Model file for the job. Use its own axes, mm. A direction names the side the tool comes from. Round coordinates to 2 decimals unless told otherwise and drop trailing zeros. Loops run counter-clockwise (first coordinate to the right, second up) from the corner with the lowest first, then second, coordinate; pieces in that order, holes last. Notation, with made-up numbers: (39, 56) -> (44, 56) arc R32 cw to (44, 90) -> close; hole circle Ø11 at (46, 29.5). An arc over 180 degrees is marked (long way). Use a Markdown table: item, result.
Autodesk Fusion 360 part; units mm, degrees
sketch "Sketch1" plane through (0, 0, 0) normal (0, 0, 1) x (1, 0, 0)
  line L0 (33, -21) -> (-33, -21)
  line L1 (-33, -21) -> (-33, 21)
  line L2 (-33, 21) -> (33, 21)
  line L3 (33, 21) -> (33, -21)
  line L4 (33, -21) -> (-33, 21) construction
  line L5 (-33, -21) -> (33, 21) construction
  dimension "d1" = 66
  dimension "d2" = 42
extrude "Extrude1" add sketch "Sketch1" along normal blind 12
chamfer "Chamfer1" distance 12 angle 45 2 edges at (33, -21, 6) (33, 21, 6)
sketch "Sketch2" plane through (0, 0, 12) normal (0, 0, 1) x (-1, 0, 0)
  line L0 (-33, -9) -> (-21, -21)
  line L1 (-21, -21) -> (33, -21)
  line L2 (33, -21) -> (33, 21)
  line L3 (33, 21) -> (-21, 21)
  line L4 (-21, 21) -> (-33, 9)
  line L5 (-33, 9) -> (-33, -9)
  line L6 (33, -21) -> (21, -21)
  line L7 (21, -21) -> (21, 21)
  line L8 (21, 21) -> (33, 21)
  line L9 (33, 21) -> (33, -21)
  dimension "d6" = 12
extrude "Extrude2" add sketch "Sketch2" along normal blind 48 contours L1 L2 L3 L6 L7 L8 L9
fillet "Fillet1" radius 21 2 edges at (-27, -21, 60) (-27, 21, 60)
sketch "Sketch3" plane through (0, 0, 0) normal (0, 1, 0) x (1, 0, 0)
  line L0 (-21.0863, -54.0506) -> (-21.0863, -12.0506)
  line L1 (-21.0863, -12.0506) -> (32.9137, -12.0506)
  line L2 (32.9137, -12.0506) -> (-21.0863, -54.0506)
  dimension "d11" = 42
  dimension "d12" = 54
extrude "Extrude3" add sketch "Sketch3" along normal mid plane 12
equation "d7 = 60 mm - 12 mm"
equation "d12 = 66 mm - 12 mm"
Q1. Flat gauge pins, fed straight in: pin 1 (3 mm diameter, centred on y = 7, z = 35.5, fed in from +X); pin 2 (12.5 mm diameter, centred on x = 13.5, z = 26, fed in from +Y); pin 3 (3 mm diameter, centred on y = -15.5, z = 19.5, fed in from +X). Where does each tip first touch, or does it go through?
Results list:
| item | result |
|---|---|
| pin 1 | stops at x = 4.2 |
| pin 2 | stops at y = 6 |
| pin 3 | stops at x = -21 |
Q2. Band-saw the part on A-A, the plane x = 22.5. Give the cut face in (y, z).
Results list:
| item | result |
|---|---|
| outline | (-19.5, 0) -> (19.5, 0) -> (19.5, 12) -> (-19.5, 12) -> close; (-6, 12.05) -> (6, 12.05) -> (6, 20.15) -> (-6, 20.15) -> close |
Q3. Band-saw the part on C-C, the plane y = 3. Give the cut face in (x, z), plus the area to 3 significant figures.
Results list:
| item | result |
|---|---|
| outline | (-33, 0) -> (33, 0) -> (33, 12) -> (-21, 12) -> (-21, 12.05) -> (32.91, 12.05) -> (-21, 53.98) -> (-21, 59.79) -> (-33, 59.79) -> close |
| area | 2,500 mm² |
Q4. Drill centre lines: L1, parallel to X at y = -15.5, z = 16; L2, parallel to Y at x = 13, z = 21; L3, parallel to Z at x = 10, y = -17. Where is each one in solid material? Low to high. Write a range as from..to.
Results list:
| item | result |
|---|---|
| L1 | x = -33..-21 |
| L2 | y = -6..6 |
| L3 | z = 0..12 |
Q5. Band-saw the part on D-D, the plane x = -13.5. Give the cut face in (y, z), plus the area to 3 significant figures.
Results list:
| item | result |
|---|---|
| outline | (-21, 0) -> (21, 0) -> (21, 12) -> (-21, 12) -> close; (-6, 12.05) -> (6, 12.05) -> (6, 48.15) -> (-6, 48.15) -> close |
| area | 937 mm² |
Q6. Band-saw the part on B-B, the plane z = 5. Give the cut face in (x, y), plus the area to 3 significant figures.
Results list:
| item | result |
|---|---|
| outline | (-33, -21) -> (21, -21) -> (33, -9) -> (33, 9) -> (21, 21) -> (-33, 21) -> close |
| area | 2,630 mm² |
Q7. Tool access for faces 1 (the face through (-12, -21, 11)), 2 (the face through (0, 6, 28)), 3 (the face through (0, -6, 28)): list every direction of +Z, -Z, +X, -X, +Y, -Y with a clear straight run to the whole face (end or side of a thin tool).
Results list:
| item | result |
|---|---|
| face 1 | +Z, -Z, +X, -X, -Y |
| face 2 | +Z, +X, +Y |
| face 3 | +Z, +X, -Y |
